CAD build for the part. Positions are in the model's coordinates, mm. Coordinates: 2 decimals unless noted, no trailing zeros. Loops run counter-clockwise (first coordinate to the right, second up) from the corner with the lowest first, then second, coordinate; pieces in that order, holes last. Notation, with made-up numbers: (35.5, -12.75) -> (63.5, -12.75) arc R20 ccw to (63.5, -7.75) -> close; hole circle Ø10 at (48.5, 29). An arc over 180 degrees is marked (long way). Write each question's results on one line, items separated by ' | '.
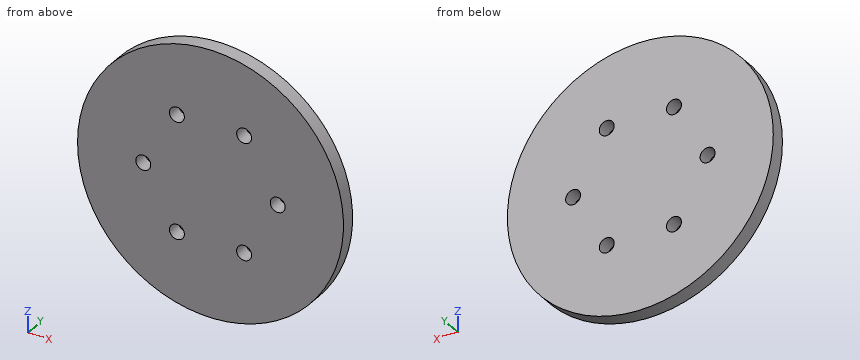
Autodesk Inventor part; units mm, degrees
ref_plane "YZ Plane" through (0, 0, 0) normal (1, 0, 0) x (0, 1, 0)
ref_plane "XZ Plane" through (0, 0, 0) normal (0, 1, 0) x (-1, 0, 0)
ref_plane "XY Plane" through (0, 0, 0) normal (0, 0, 1) x (1, 0, 0)
sketch "Sketch1" plane through (0, 0, 0) normal (0, 1, 0) x (-1, 0, 0)
  circle A0 centre (0, 0) radius 8.9
  dimension "d0" = 17.8
extrude "Extrusion1" add sketch "Sketch1" along normal blind 1
sketch "Sketch2" plane through (0, 1, 0) normal (0, 1, 0) x (1, 0, 0)
  point P0 (0, 0)
  point P1 (-4.5, 0)
  dimension "d4" = 4.5
hole "Hole1" at (-4.5, 1, 0) direction (0, -1, 0) diameter 1 end through all
pattern_circular "Circular Pattern1" count 6 over 360 about axis through (0, 0, 0) along (0, 1, 0) of "Hole1"
properties part number "EpoxyFitThroughKF16_mask" material "Epoxy Resin"
Q1. Wall check: L1, parallel to X at y = 0.85, z = -3.5; L2, parallel to Z at x = 4.75, y = 0.15; L3, parallel to X at y = 0.2, z = -3. Give the ranges that are in metal, low to high. Write a range as from..to.
Results are:
L1: -8.18..-2.55, -1.95..1.95, 2.55..8.18 | L2: -7.53..-0.43, 0.43..7.53 | L3: -8.38..8.38
Q2. Drop a flat-ended pin along its axis: pin 1 (2 mm diameter, centred on x = -2.5, z = 6, fed in from -Y). Give the stop position or say it passes through.
Results are:
pin 1: y = 0
Q3. Cut at B-B on x = 4.5. Write the cut outline in (y, z), and give its area (3 significant figures).
Results are:
outline: (0, -7.68) -> (1, -7.68) -> (1, -0.5) -> (0, -0.5) -> close; (0, 0.5) -> (1, 0.5) -> (1, 7.68) -> (0, 7.68) -> close | area: 14.4 mm^2
Q4. Cut at C-C on y = 0.85. Write the cut outline in (x, z).
Results are:
outline: circle Ø17.8 at (0, 0); hole circle Ø1 at (-4.5, 0); hole circle Ø1 at (-2.25, -3.9); hole circle Ø1 at (-2.25, 3.9); hole circle Ø1 at (2.25, -3.9); hole circle Ø1 at (2.25, 3.9); hole circle Ø1 at (4.5, 0)
Q5. Cut at A-A on z = 0. Write the cut outline in (x, y).
Results are:
outline: (-8.9, 0) -> (-5, 0) -> (-5, 1) -> (-8.9, 1) -> close; (-4, 0) -> (4, 0) -> (4, 1) -> (-4, 1) -> close; (5, 0) -> (8.9, 0) -> (8.9, 1) -> (5, 1) -> close
Q6. Cut at D-D on x = 2.25. Write the cut outline in (y, z).
Results are:
outline: (0, -8.61) -> (1, -8.61) -> (1, -4.4) -> (0, -4.4) -> close; (0, -3.4) -> (1, -3.4) -> (1, 3.4) -> (0, 3.4) -> close; (0, 4.4) -> (1, 4.4) -> (1, 8.61) -> (0, 8.61) -> close
